from build123d import *

# Parameters (mm, degrees)
BOSS_EXTRUDE1_DEPTH = 6.35
CUT_EXTRUDE1_DEPTH  = 6.35
SKETCH4_R           = 2
SKETCH4_W           = 6.35
SKETCH4_H           = 12.7
CUT_EXTRUDE5_DEPTH  = 6.35
SKETCH6_W           = 6.35
SKETCH6_H           = 12.7
CUT_EXTRUDE6_DEPTH  = 6.35
CUT_EXTRUDE7_DEPTH  = 6.35
SKETCH5_W           = 6.35
SKETCH5_H           = 12.7
CUT_EXTRUDE4_DEPTH  = 6.35


with BuildPart() as part:
    # Sketch1 → Boss-Extrude1 (new body)
    with BuildSketch(Plane.XY):
        Polygon((190.5, 508), (120.65, 508), (0, 25.4), (0, 6.35), (19.05, 6.35), (19.05, 0), (31.75, 0), (31.75, 6.35), (82.55, 6.35), (82.55, 0), (95.25, 0), (95.25, 6.35), (133.35, 6.35), (133.35, 0), (146.05, 0), (146.05, 6.35), (158.75, 6.35), (158.75, 0), (190.5, 0), (196.85, 0), (196.85, 508), align=None)
        Polygon((120.65, 50.8), (120.65, 403.273117109), (82.55, 250.873117109), (82.55, 50.8), align=None, mode=Mode.SUBTRACT)
    extrude(amount=BOSS_EXTRUDE1_DEPTH)

    # Sketch2 → Cut-Extrude1 (cut)
    with BuildSketch(Plane.XY.offset(6.35)):
        Polygon((59.53125, 6.35), (54.76875, 6.35), (54.76875, 14.2875), (52.3875, 14.2875), (52.3875, 17.4625), (54.76875, 17.4625), (54.76875, 20.6375), (59.53125, 20.6375), (59.53125, 17.4625), (61.9125, 17.4625), (61.9125, 14.2875), (59.53125, 14.2875), align=None)
        Polygon((116.68125, 6.35), (111.91875, 6.35), (111.91875, 14.2875), (109.5375, 14.2875), (109.5375, 17.4625), (111.91875, 17.4625), (111.91875, 20.6375), (116.68125, 20.6375), (116.68125, 17.4625), (119.0625, 17.4625), (119.0625, 14.2875), (116.68125, 14.2875), align=None)
    extrude(amount=-CUT_EXTRUDE1_DEPTH, mode=Mode.SUBTRACT)

    # Sketch4 → Cut-Extrude5 (cut)
    with BuildSketch(Plane.XY.offset(6.35)):
        with Locations((130.175, 127)):
            Circle(SKETCH4_R)
        with Locations((130.175, 381)):
            Circle(SKETCH4_R)
        with Locations((130.175, 196.85)):
            Rectangle(SKETCH4_W, SKETCH4_H)
        with Locations((130.175, 57.15)):
            Rectangle(SKETCH4_W, SKETCH4_H)
        with Locations((130.175, 450.85)):
            Rectangle(SKETCH4_W, SKETCH4_H)
        with Locations((130.175, 311.15)):
            Rectangle(SKETCH4_W, SKETCH4_H)
    extrude(amount=-CUT_EXTRUDE5_DEPTH, mode=Mode.SUBTRACT)

    # Sketch6 → Cut-Extrude6 (cut)
    with BuildSketch(Plane.XY.offset(6.35)):
        with Locations((60.325, 44.45)):
            Rectangle(SKETCH6_W, SKETCH6_H)
    extrude(amount=-CUT_EXTRUDE6_DEPTH, mode=Mode.SUBTRACT)

    # Sketch7 → Cut-Extrude7 (cut)
    with BuildSketch(Plane.XY.offset(6.35)):
        Polygon((82.55, 50.8), (69.85, 50.8), (69.85, 200.073117109), (82.55, 250.873117109), align=None)
    extrude(amount=-CUT_EXTRUDE7_DEPTH, mode=Mode.SUBTRACT)

    # Sketch5 → Cut-Extrude4 (cut)
    with BuildSketch(Plane.XY.offset(6.35)):
        with Locations((54.590058309, 44.45)):
            Rectangle(SKETCH5_W, SKETCH5_H)
    extrude(amount=-CUT_EXTRUDE4_DEPTH, mode=Mode.SUBTRACT)


solid = part.part
Could you check a few things on this model? Use its own coordinates, in mm. A direction names the side the tool comes from. Give positions to 0.01 mm unless a question says otherwise; leave off trailing zeros. Write each loop counter-clockwise with the first axis right and the second up, starting at its lowest first coordinate (ties: lowest second). Pieces come first, ordered by that corner, then holes. Notation, with made-up numbers: (-11, 32) -> (21, 32) arc R14 cw to (21, 49) -> close; hole circle Ø5 at (69, 28.25). An arc over 180 degrees is marked (long way). Answer as CSV lines item,"result". Start each with the question number.
(1) If we section it at D-D, the plane y = 473.5: Write out the boundary of the cut face in (x, z) (3 decimals).
(2) If we section it at B-B, the plane x = 103.5: Write out the boundary of the cut face in (y, z), and give its area (3 significant figures).
(3) If we section it at C-C, the plane z = 2.75: Give the number of separate pieces and of enclosed holes in the cut face, and give its area (3 significant figures).
(4) I'm going to push flat-ended pins straight in: pin 1 Ø1.5 at (x, z) = (126, 2) entering from -Y; pin 2 Ø4.5 at (x, y) = (130.175, 127) entering from -Z; pin 3 Ø1.9 at (y, z) = (4.5, 2) entering from -X; pin 4 Ø1.4 at (x, z) = (115, 2.5) entering from -Y. Where does each tip first touch, or does it pass through?
(5) Which directions (+Z, -Z, +X, -X, +Y, -Y) give clear straight access to the entire face, cutting with the end or side of a thin tool? Please do faces 1 (the face through (95.606, 303.096, 3.131)), 2 (the face through (141, 201, 0)).
(6) If we section it at A-A, the plane y = 115: Write out the boundary of the cut face in (x, z), and give its area (3 significant figures).
(7) Please list where these lines run through material, in increasing order: line 1 (X direction, y = 381, z = 4.25) (3 decimals); line 2 (X direction, y = 194, z = 1.5); line 3 (X direction, y = 140, z = 5.5).
Answer list:
1,outline,"(112.025, 0) -> (196.85, 0) -> (196.85, 6.35) -> (112.025, 6.35) -> close"
2,outline,"(6.35, 0) -> (50.8, 0) -> (50.8, 6.35) -> (6.35, 6.35) -> close; (334.67, 0) -> (439.4, 0) -> (439.4, 6.35) -> (334.67, 6.35) -> close"
2,area,"947 mm^2"
3,separate pieces,"1"
3,enclosed holes,"8"
3,area,"56,700 mm^2"
4,pin 1,"y = 6.35"
4,pin 2,"z = 0"
4,pin 3,"x = 19.05"
4,pin 4,"y = 20.64"
5,face 1,"+Z, -Z"
5,face 2,"-Z, +X, -X, +Y, -Y"
6,outline,"(22.4, 0) -> (69.85, 0) -> (69.85, 6.35) -> (22.4, 6.35) -> close; (120.65, 0) -> (196.85, 0) -> (196.85, 6.35) -> (120.65, 6.35) -> close"
6,area,"785 mm^2"
7,line 1,"88.9 to 115.082, 120.65 to 128.175, 132.175 to 196.85"
7,line 2,"42.15 to 69.85, 120.65 to 127, 133.35 to 196.85"
7,line 3,"28.65 to 69.85, 120.65 to 196.85"
